Design review of the part built by this model. Coordinates are the model's own, in mm. A direction names the side the tool comes from. Coordinates: 2 decimals unless noted, no trailing zeros. Order: outer loops, then holes, each group sorted by start corner. A loop starts at its lowest first (then second) coordinate and runs counter-clockwise, first axis right, second up. Notation, with made-up numbers: M -34.75,34 L -26.75,34 A17 ccw -26.75,66 Z; hole C 67.25,5.25 d8. An arc over 180 degrees is marked long. Use CSV: the item, a comma, the result in double quotes.
```python
from build123d import *

# Parameters (mm, degrees)
F1_DEPTH  = 10
F3_DEPTH  = 10.001
F5_DEPTH  = 25
F6_R      = 1.395
F7_DEPTH  = 25
F8_R      = 4.25
F9_DEPTH  = 112.584302492
F8_R_2    = 5.6
F10_DEPTH = 1.5


with BuildPart() as f1:
    # F0 (on Front) → F1 (new body, symmetric)
    with BuildSketch(Plane.XZ):
        with BuildLine():
            Line((30, 51.9615242271), (0, 0))
            Line((0, 0), (130, 0))
            Line((130, 0), (130, 10))
            Line((130, 10), (88.0384757729, 10))
            ThreePointArc((88.0384757729, 10), (82.8620948709, 10.6814834742), (78.0384757729, 12.6794919243))
            Line((78.0384757729, 12.6794919243), (62.2390923627, 21.8012701892))
            ThreePointArc((62.2390923627, 21.8012701892), (61.5402036233, 22.7120797272), (61.6900542571, 23.8503082949))
            Line((61.6900542571, 23.8503082949), (62.1900542571, 24.7163336987))
            Line((62.1900542571, 24.7163336987), (44.8695461814, 34.7163336987))
            Line((44.8695461814, 34.7163336987), (44.3695461814, 33.8503082949))
            ThreePointArc((44.3695461814, 33.8503082949), (43.4587366433, 33.1514195555), (42.3205080757, 33.3012701892))
            Line((42.3205080757, 33.3012701892), (27.5980762114, 41.8012701892))
            ThreePointArc((27.5980762114, 41.8012701892), (26.8991874719, 42.7120797272), (27.0490381057, 43.8503082949))
            Line((27.0490381057, 43.8503082949), (31.2990381057, 51.2115242271))
            Line((31.2990381057, 51.2115242271), (30, 51.9615242271))
        make_face()
        with BuildLine():
            Line((27.4019237886, 1.5), (13.1291651246, 9.7403810568))
            ThreePointArc((13.1291651246, 9.7403810568), (10.7995359932, 12.7764128502), (11.2990381057, 16.5705080757))
            Line((11.2990381057, 16.5705080757), (23.0490381057, 36.9221050646))
            ThreePointArc((23.0490381057, 36.9221050646), (26.0850698991, 39.2517341961), (29.8791651246, 38.7522320835))
            Line((29.8791651246, 38.7522320835), (78.2416697508, 10.8301270189))
            ThreePointArc((78.2416697508, 10.8301270189), (80.5712988822, 5.2059047745), (75.7416697508, 1.5))
            Line((75.7416697508, 1.5), (27.4019237886, 1.5))
        make_face(mode=Mode.SUBTRACT)
    extrude(amount=F1_DEPTH, both=True)

    # F2 (on face) → F3 (cut, through all)
    with BuildSketch(Plane.XY.offset(10)):
        with BuildLine():
            Line((130, 3), (113, 3))
            ThreePointArc((113, 3), (110, 0), (113, -3))
            Line((113, -3), (130, -3))
            Line((130, -3), (130, 3))
        make_face()
        with BuildLine():
            Line((98, 5), (130, 5))
            Line((130, 5), (130, 10))
            Line((130, 10), (95, 10))
            Line((95, 10), (95, 8))
            ThreePointArc((95, 8), (95.8786796564, 5.8786796564), (98, 5))
        make_face()
        with BuildLine():
            Line((95, -10), (130, -10))
            Line((130, -10), (130, -5))
            Line((130, -5), (98, -5))
            ThreePointArc((98, -5), (95.8786796564, -5.8786796564), (95, -8))
            Line((95, -8), (95, -10))
        make_face()
    extrude(amount=-F3_DEPTH, mode=Mode.SUBTRACT)

    # F4 (on face) → F5 (cut)
    with BuildSketch(Plane(origin=(30, 0, 51.9615242271), x_dir=(0.8660254038, 0, -0.5), z_dir=(0.5, 0, 0.8660254038))):
        with BuildLine():
            ThreePointArc((28, 4), (24, 0), (28, -4))
            Line((28, -4), (35, -4))
            ThreePointArc((35, -4), (39, 0), (35, 4))
            Line((35, 4), (28, 4))
        make_face()
    extrude(amount=-F5_DEPTH, mode=Mode.SUBTRACT)

    # F6 (on face) → F7 (cut)
    with BuildSketch(Plane(origin=(0, 0, 0), x_dir=(0, -1, 0), z_dir=(-0.8660254038, 0, 0.5))):
        with Locations((-5, 25)):
            Circle(F6_R)
        with Locations((-5, 32)):
            Circle(F6_R)
        with Locations((-5, 39)):
            Circle(F6_R)
        with Locations((5, 25)):
            Circle(F6_R)
        with Locations((5, 32)):
            Circle(F6_R)
        with Locations((5, 39)):
            Circle(F6_R)
    extrude(amount=-F7_DEPTH, mode=Mode.SUBTRACT)

    # F8 (on face) → F9 (cut, through all)
    with BuildSketch(Plane(origin=(0, 0, 0), x_dir=(0, -1, 0), z_dir=(-0.8660254038, 0, 0.5))):
        with Locations((0, 7.5)):
            Circle(F8_R)
    extrude(amount=-F9_DEPTH, mode=Mode.SUBTRACT)

    # F8 (on face) → F10 (cut)
    with BuildSketch(Plane(origin=(0, 0, 0), x_dir=(0, -1, 0), z_dir=(-0.8660254038, 0, 0.5))):
        with Locations((0, 7.5)):
            Circle(F8_R_2)
        with Locations((0, 7.5)):
            Circle(F8_R, mode=Mode.SUBTRACT)
    extrude(amount=-F10_DEPTH, mode=Mode.SUBTRACT)


solid = f1.part
```
(1) Add section C-C on x = 37.5. State the section outline as (y, z) points, and give its area (3 significant figures).
The answers:
outline,"M -10,0 L 10,0 L 10,1.5 L -10,1.5 Z; M -10,34.35 L 10,34.35 L 10,36.08 L -10,36.08 Z"
area,"64.6 mm2"
(2) For faces 1 (the face through (29.144, -0.14, 47.479)), 2 (the face through (53.7, -4.6, 25)), 3 (the face through (114, 5, 5)), list the 3-axis set-ups (+Z, -Z, +X, -X, +Y, -Y) from which the entire face can be reached by the end or side of a thin tool; tool diameter is ignored.
The answers:
face 1,"+X, +Y, -Y"
face 2,"+Y, -Y"
face 3,"+Z, -Z, +X, +Y"
(3) Wall thickness on probe 1 along X at (y, z) = (5.25, 35); probe 2 along X at (y, z) = (3.75, 12.5); probe 3 along Z at (x, y) = (23, 0.75): over which ranges is each line inside the solid? List them lowest first.
The answers:
probe 1,"x = 20.21 to 21.94, 36.38 to 39.38"
probe 2,"x = 7.22 to 10.88, 75.35 to 78.36"
probe 3,"z = 0.21 to 4.04, 36.84 to 39.84"
(4) The part is to be moulded in two halves that separate along Z. For faces 4 (the face through (64, 0, 0)), 5 (the face through (95.86, 5.9, 5.07)), 6 (the face through (17.09, -0.14, 26.6)), say which applies: pulls with the +Z half, pulls with the -Z half, needs draft (parallel to the pull), parting line crosses it, or undercut.
The answers:
face 4,"pulls with the -Z half"
face 5,"needs draft"
face 6,"undercut"
(5) Add section A-A on x = 117.5. State the section outline as (y, z) points.
The answers:
outline,"M -5,0 L -3,0 L -3,10 L -5,10 Z; M 3,0 L 5,0 L 5,10 L 3,10 Z"
(6) Add section D-D on x = 90.5. State the section outline as (y, z) points, and give its area (3 significant figures).
The answers:
outline,"M -10,0 L 10,0 L 10,10 L -10,10 Z"
area,"200 mm2"
(7) Clearance check with flat-ended pins moving along their axes: P1, Ø12, axis at y = -7.5, z = 15.5, coming from the -X side; P2, Ø2, axis at y = 1.5, z = 36, coming from the +X side; P3, Ø0.6, axis at y = -9, z = 3.5, coming from the +X side; P4, Ø3, axis at x = 18, z = 22.5, coming from the -Y side. State where each tip first meets the part, or that it passes through.
The answers:
P1,"stops at x = 5.48"
P2,"stops at x = 39.38"
P3,"stops at x = 95"
P4,"passes through"
